Can you work these out from the model? Positions are in its coordinate system, mm. Face numbers are marked on the shaded views. Round coordinates to 2 decimals unless told otherwise and drop trailing zeros. Loops run counter-clockwise (first coordinate to the right, second up) from the corner with the lowest first, then second, coordinate; pieces in that order, holes last.
(1) Will these pins go through, and if not, where does the flat tip stop? pin 1 Ø4 at (y, z) = (-29.5, 20.5) entering from -X; pin 2 Ø4 at (x, y) = (-72, -20) entering from +Z; pin 3 Ø1.9 at (x, z) = (-46.5, 3) entering from -Y.
(2) If I drill on line 1 along Y through (x, z) = (0, 15.25); line 2 along X through (y, z) = (-1, 7.5); line 3 along Z through (x, y) = (-54, -16.5), over which ranges is the centre line in solid material (lowest first)?
(3) Thinking about a two-plate mould opening in X: for the marked faces 1, 2 and 3, which applies, released by +X, released by -X, zero draft, split by the parting line, or undercut?
(4) I want a section at C-C on y = -9. Write out the boundary of the cut face in (x, z).
(5) I want a section at D-D on y = 29. Write out the boundary of the cut face in (x, z).
(6) I want a section at A-A on z = 14. Write out the boundary of the cut face in (x, y).
(7) I want a section at B-B on x = -2. Write out the boundary of the cut face in (y, z), plus the area to 3 significant figures.
from build123d import *

# Parameters (mm, degrees)
F1_DEPTH      = 6.35
F0_R          = 25.4
F2_DEPTH      = 25.4
F4_DEPTH      = 6.35
F4_DEPTH_BACK = 6.35


with BuildPart() as f1:
    # F0 (on Top) → F1 (new body)
    with BuildSketch(Plane.XY):
        with BuildLine():
            ThreePointArc((-21.060567, -31.75), (-38.1, 0), (-21.060567, 31.75))
            Line((-21.060567, 31.75), (-88.9, 31.75))
            Line((-88.9, 31.75), (-88.9, -31.75))
            Line((-88.9, -31.75), (-21.060567, -31.75))
        make_face()
    extrude(amount=F1_DEPTH)

    # F0 (on Top) → F2 (join)
    with BuildSketch(Plane.XY):
        with BuildLine():
            ThreePointArc((-21.060567, -31.75), (18.016692, -33.570952), (38.1, 0))
            ThreePointArc((38.1, 0), (18.016692, 33.570952), (-21.060567, 31.75))
            ThreePointArc((-21.060567, 31.75), (-38.1, 0), (-21.060567, -31.75))
        make_face()
        Circle(F0_R, mode=Mode.SUBTRACT)
    extrude(amount=F2_DEPTH)

    # F3 (on Front) → F4 (join, two sides)
    with BuildSketch(Plane.XZ) as f4_sk:
        Polygon((-82.73942, 3.131038), (-38.28942, 3.131038), (-38.28942, 22.181038), align=None)
    extrude(amount=F4_DEPTH)
    extrude(f4_sk.sketch, amount=-F4_DEPTH_BACK)


solid = f1.part
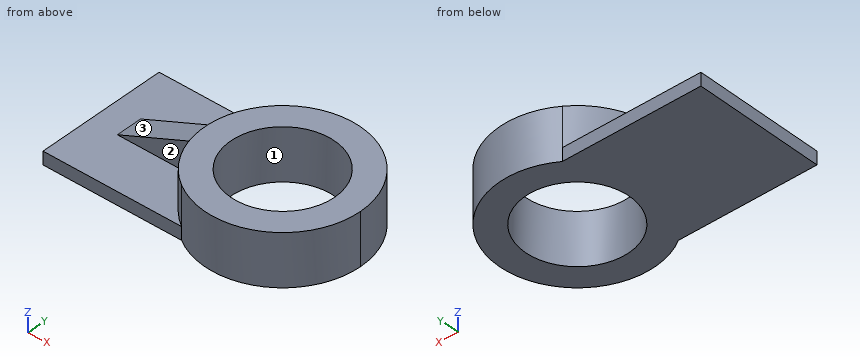
Filled sheet:
1. pin 1: stops at x = -26.37
1. pin 2: stops at z = 6.35
1. pin 3: stops at y = -31.75
2. line 1: y = -38.1 to -25.4, 25.4 to 38.1
2. line 2: x = -72.55 to -38.29, -38.09 to -25.38, 25.38 to 38.09
2. line 3: z = 0 to 6.35
3. face 1: undercut
3. face 2: zero draft
3. face 3: released by -X
4. outline: (-88.9, 0) - (-23.75, 0) - (-23.75, 25.4) - (-37.02, 25.4) - (-37.02, 6.35) - (-88.9, 6.35) - close; (23.75, 0) - (37.02, 0) - (37.02, 25.4) - (23.75, 25.4) - close
5. outline: (-88.9, 0) - (24.71, 0) - (24.71, 25.4) - (-24.71, 25.4) - (-24.71, 6.35) - (-88.9, 6.35) - close
6. outline: (-57.38, -6.35) - (-38.29, -6.35) - (-38.29, 6.35) - (-57.38, 6.35) - close; circle Ø76.2 at (0, 0); hole circle Ø50.8 at (0, 0)
7. outline: (-38.05, 0) - (-25.32, 0) - (-25.32, 25.4) - (-38.05, 25.4) - close; (25.32, 0) - (38.05, 0) - (38.05, 25.4) - (25.32, 25.4) - close
7. area: 646 mm2
